```python
from build123d import *

# Parameters (mm, degrees)
SKETCH1_R           = 16
BOSS_EXTRUDE1_DEPTH = 3
SKETCH3_R           = 1
BOSS_EXTRUDE2_DEPTH = 3
SKETCH4_R           = 10
BOSS_EXTRUDE3_DEPTH = 15
CUT_EXTRUDE1_REACH  = 29.148
SKETCH5_R           = 9
FILLET1_R           = 1
FILLET2_R           = 0.5


with BuildPart() as part:
    # Sketch1 → Boss-Extrude1 (new body)
    with BuildSketch(Plane(origin=(0, 0, 0), x_dir=(1, 0, 0), z_dir=(0, 1, 0))):
        with Locations(Location((0, 0, 0), (0, 0, 270))):
            Circle(SKETCH1_R)
        with BuildLine():
            Line((2.645751311, 3), (8, 3))
            Line((8, 3), (8, -3))
            Line((8, -3), (2.645751311, -3))
            ThreePointArc((2.645751311, -3), (0, -4), (-2.645751311, -3))
            Line((-2.645751311, -3), (-8, -3))
            Line((-8, -3), (-8, 3))
            Line((-8, 3), (-2.645751311, 3))
            ThreePointArc((-2.645751311, 3), (0, 4), (2.645751311, 3))
        make_face(mode=Mode.SUBTRACT)
    extrude(amount=BOSS_EXTRUDE1_DEPTH)

    # Sketch3 → Boss-Extrude2 (add)
    with BuildSketch(Plane.XZ):
        with Locations(Location((-13, 0, 0), (0, 0, 90))):
            Circle(SKETCH3_R)
    extrude(amount=BOSS_EXTRUDE2_DEPTH)

    # Sketch4 → Boss-Extrude3 (add)
    with BuildSketch(Plane.XZ):
        with Locations(Location((0, 0, 0), (0, 0, 90))):
            Circle(SKETCH4_R)
    extrude(amount=BOSS_EXTRUDE3_DEPTH)

    # Sketch5 → Cut-Extrude1 (cut, up to next)
    with BuildSketch(Plane(origin=(0, 0, 0), x_dir=(1, 0, 0), z_dir=(0, 1, 0)), mode=Mode.PRIVATE) as cut_extrude1_sk1:
        with Locations(Location((0, 0, 0), (0, 0, 270))):
            Circle(SKETCH5_R)
    cut_extrude1_tool1 = extrude(cut_extrude1_sk1.sketch, amount=-CUT_EXTRUDE1_REACH, mode=Mode.PRIVATE) & part.part
    add(cut_extrude1_tool1.solids().sort_by_distance((0, 0, 0))[0], mode=Mode.SUBTRACT)

    # Fillet1
    fillet1_edges = [part.edges().sort_by_distance(p)[0] for p in [
        (0, -15, -10),
    ]]
    fillet(fillet1_edges, radius=FILLET1_R - 0.0001)  # a hair under: the kernel refuses the full size

    # Fillet2
    fillet2_edges = [part.edges().sort_by_distance(p)[0] for p in [
        (0, 0, -16),
        (0, 3, -16),
    ]]
    fillet(fillet2_edges, radius=FILLET2_R)


solid = part.part
```
Could you check a few things on this model? Use its own coordinates, in mm. A direction names the side the tool comes from. Coordinates: 2 decimals unless noted, no trailing zeros. Write each loop counter-clockwise with the first axis right and the second up, starting at its lowest first coordinate (ties: lowest second). Pieces come first, ordered by that corner, then holes. Notation, with made-up numbers: (9, 8.25) -> (57, 8.25) arc R13 ccw to (57, 24.25) -> close; hole circle Ø4 at (46.25, -23). An arc over 180 degrees is marked (long way). Return JSON: item names as keys, results as strings.
(1) Imagine slicing it at D-D, the plane y = -8.5. Please give me the cut outline in (x, z), then the cut area to 3 significant figures.
Numbers:
{"outline": "circle Ø20 at (0, 0); hole circle Ø18 at (0, 0)", "area": "59.7 mm2"}
(2) Imagine slicing it at B-B, the plane y = 1.5. Please give me the cut outline in (x, z).
Numbers:
{"outline": "circle Ø32 at (0, 0); hole (-8, -3) -> (-2.65, -3) arc R4 ccw to (2.65, -3) -> (8, -3) -> (8, 3) -> (2.65, 3) arc R4 ccw to (-2.65, 3) -> (-8, 3) -> close"}
(3) We'd pull the mould along Z, two halves only. Please class faces 4 (the flat face through (-13, -3, 0)), 5 (the cylindrical face through (9.76, -6.9, -2.17)), 6 (the flat face through (8, 1, 0)): +Z half, -Z half, draft (parallel to the pull), parting line (faces both ways), or undercut.
Numbers:
{"face 4": "draft", "face 5": "parting line", "face 6": "undercut"}
(4) Which directions (+Z, -Z, +X, -X, +Y, -Y) give clear straight access to the entire face, cutting with the end or side of a thin tool? Please do faces 1 (the flat face through (5, 1, 3)), 2 (the cylindrical face through (-12, -1, 0)), 3 (the flat face through (-3.2, 3, 3.2)).
Numbers:
{"face 1": "+Y, -Y", "face 2": "-Y", "face 3": "+Z, -Z, +X, -X, +Y"}
(5) I need wall thicknesses on L1, parallel to X at y = -7.75, z = 0; L2, parallel to Y at x = -4, z = 10.5; L3, parallel to Z at x = 6, y = -2.5. Which ranges of each line are inside material? Lowest first, please.
Numbers:
{"L1": "x = -10 to -9, 9 to 10", "L2": "y = 0 to 3", "L3": "z = -8 to -6.71, 6.71 to 8"}
(6) I'm going to push flat-ended pins straight in: pin 1 (16 mm diameter, centred on x = 0, z = 0, fed in from -Y); pin 2 (6 mm diameter, centred on y = -0.5, z = -10, fed in from -X); pin 3 (0.6 mm diameter, centred on x = -13.5, z = 0, fed in from -Y). Where does each tip first touch, or does it pass through?
Numbers:
{"pin 1": "stops at y = 0", "pin 2": "stops at x = -14.31", "pin 3": "stops at y = -3"}
